from build123d import *

# Parameters (mm, degrees)
SKETCH_1_W          = 40
SKETCH_1_H          = 30
EXTRUDE_1_DEPTH     = 30
SKETCH_2_R          = 7.5
SKETCH_2_R_2        = 5
EXTRUDE_2_DEPTH     = 5
SKETCH_2_2_R        = 5
CUT_EXTRUDE_1_DEPTH = 40.05124838


with BuildPart() as part:
    # Эскиз1 → Бобышка-Вытянуть1 (new body)
    with BuildSketch(Plane(origin=(0, 0, 0), x_dir=(0, 0, -1), z_dir=(1, 0, 0))):
        Rectangle(SKETCH_1_W, SKETCH_1_H)
    extrude(amount=-EXTRUDE_1_DEPTH)

    # Эскиз2 → Бобышка-Вытянуть2 (add)
    with BuildSketch(Plane(origin=(0, 0, 0), x_dir=(0, 0, -1), z_dir=(1, 0, 0))):
        with Locations((5, 0)):
            Circle(SKETCH_2_R)
        with Locations((5, 0)):
            Circle(SKETCH_2_R_2, mode=Mode.SUBTRACT)
    extrude(amount=EXTRUDE_2_DEPTH)

    # Эскиз2<2> → Вырез-Вытянуть1 (cut, through all)
    with BuildSketch(Plane(origin=(0, 0, 0), x_dir=(0, 0, -1), z_dir=(1, 0, 0))):
        with Locations((5, 0)):
            Circle(SKETCH_2_2_R)
    extrude(amount=-CUT_EXTRUDE_1_DEPTH, mode=Mode.SUBTRACT)


solid = part.part
Geometry: final body of the model. Coordinates: model frame, mm. A direction names the side the tool comes from. Coordinates: 2 decimals unless noted, no trailing zeros. Order: outer loops, then holes, each group sorted by start corner. A loop starts at its lowest first (then second) coordinate and runs counter-clockwise, first axis right, second up. Notation, with made-up numbers: M 46.5,1 L 102.5,1 A27 cw 102.5,19 Z; hole C 32,-9 d8. An arc over 180 degrees is marked long. One line per question, with ' | ' between items. Start each with the question number.
Item 1: Cut plane C-C, the plane x = -25. Return the cut outline in (y, z).
Item 2: Cut plane D-D, the plane z = -13. Return the cut outline in (x, y), then the cut area to 3 significant figures.
Item 3: Ray query, probe 1 along Y at (x, z) = (-6, -5); probe 2 along Y at (x, z) = (1, -5); probe 3 along X at (y, z) = (11, -4). Return the intervals inside material, ascending. Write a range as [from, to].
Item 4: Cut plane B-B, the plane z = -5. Return the cut outline in (x, y).
Item 5: Cut plane A-A, the plane y = 0. Return the cut outline in (x, z).
Item 6: Set-up query: faces 1 (the cylindrical face through (2.46, -2.87, -11.93)), 2 (the flat face through (-15, -15, 0)). Return all of +Z, -Z, +X, -X, +Y, -Y with unobstructed straight access to the full face (end or side cutting, diameter ignored); none if empty.
Item 7: Pin query (flat end, axial travel): pin 1 Ø5 at (y, z) = (0.5, -14) entering from +X; pin 2 Ø6 at (y, z) = (0, -5) entering from -X. Return the tip coordinate at first contact, or that it passes through.
A:
1) outline: M -15,-20 L 15,-20 L 15,20 L -15,20 Z; hole C 0,-5 d10
2) outline: M -30,-15 L 0,-15 L 0,15 L -30,15 Z | area: 900 mm2
3) probe 1: y = [-15, -5], [5, 15] | probe 2: y = [-7.5, -5], [5, 7.5] | probe 3: x = [-30, 0]
4) outline: M -30,-15 L 0,-15 L 0,-7.5 L 5,-7.5 L 5,-5 L -30,-5 Z; M -30,5 L 5,5 L 5,7.5 L 0,7.5 L 0,15 L -30,15 Z
5) outline: M -30,-20 L 0,-20 L 0,-12.5 L 5,-12.5 L 5,-10 L -30,-10 Z; M -30,0 L 5,0 L 5,2.5 L 0,2.5 L 0,20 L -30,20 Z
6) face 1: +X | face 2: +Z, -Z, +X, -X, -Y
7) pin 1: stops at x = 5 | pin 2: passes through
